Work out the finished part from the listing and answer in its coordinate system (mm). Face numbers are marked on the shaded views. A direction names the side the tool comes from. Coordinates: 2 decimals unless noted, no trailing zeros. Order: outer loops, then holes, each group sorted by start corner. A loop starts at its lowest first (then second) coordinate and runs counter-clockwise, first axis right, second up. Notation, with made-up numbers: M -34,68.25 L 2,68.25 A27 cw 2,96.25 Z; hole C -28.5,12.25 d11. An arc over 180 degrees is marked long. Use a Markdown table: item, result. Add a question column.
from build123d import *

# Parameters (mm, degrees)
F4_R     = 5
F5_DEPTH = 2.5


with BuildPart() as f2:
    # F2: sweep along a path in F0
    with BuildLine(Plane.XY) as f2_path:
        Line((0, 60), (-90, 60))
        ThreePointArc((-90, 60), (-97.0710678119, 57.0710678119), (-100, 50))
        Line((-100, 50), (-100, 0))
    # F1 (on Right) → F2 (sweep)
    with BuildSketch(Plane.YZ):
        with BuildLine():
            Line((95.0018057663, -9.8656333278), (100, -10))
            Line((100, -10), (100, 10))
            Line((100, 10), (95, 10))
            Line((95, 10), (95, 5.5))
            ThreePointArc((95, 5.5), (94.1213203436, 3.3786796564), (92, 2.5))
            Line((92, 2.5), (68, 2.5))
            ThreePointArc((68, 2.5), (65.8786796564, 3.3786796564), (65, 5.5))
            Line((65, 5.5), (65, 10))
            Line((65, 10), (60, 10))
            Line((60, 10), (60, 0))
            Line((60, 0), (60, -10))
            Line((60, -10), (65, -10))
            Line((65, -10), (65, -5.5))
            ThreePointArc((65, -5.5), (65.8786796564, -3.3786796564), (68, -2.5))
            Line((68, -2.5), (92.0018057663, -2.5))
            ThreePointArc((92.0018057663, -2.5), (94.1231261099, -3.3786796564), (95.0018057663, -5.5))
            Line((95.0018057663, -5.5), (95.0018057663, -9.8656333278))
        make_face()
    sweep(path=f2_path.line)

    # F3: F2 across plane


with BuildPart() as f2_1:
    add(f2.part)
    add(f2.part.mirror(Plane.XZ))

    # F4 (on Top) → F5 (join, symmetric)
    with BuildSketch(Plane.XY):
        with BuildLine():
            Line((-70, 100), (0, 100))
            Line((0, 100), (0, 130))
            ThreePointArc((0, 130), (-13.3277028936, 148.8541892248), (-35.5480451324, 142.5800752207))
            Line((-35.5480451324, 142.5800752207), (-70, 100))
        make_face()
        with Locations((-20, 130)):
            Circle(F4_R, mode=Mode.SUBTRACT)
        with BuildLine():
            Line((0, -130), (0, -100))
            Line((0, -100), (-70, -100))
            Line((-70, -100), (-35.5480451324, -142.5800752207))
            ThreePointArc((-35.5480451324, -142.5800752207), (-13.3277028936, -148.8541892248), (0, -130))
        make_face()
        with Locations((-20, -130)):
            Circle(F4_R, mode=Mode.SUBTRACT)
    extrude(amount=F5_DEPTH, both=True)


solid = f2_1.part
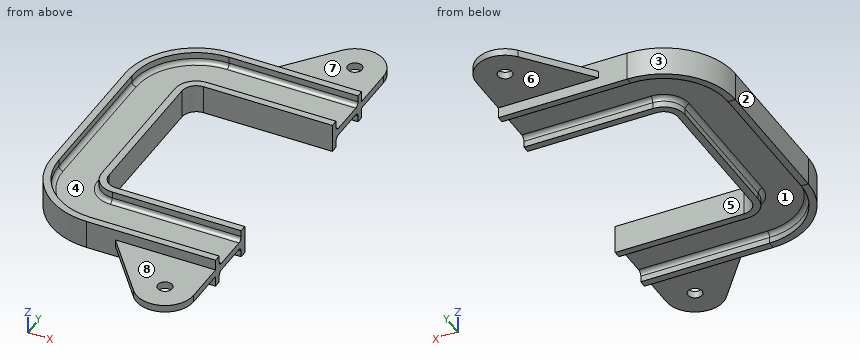
(1) Straight lines are drawn through the part: line 1 (Y direction, x = -79, z = 6); line 2 (Y direction, x = -20, z = -0.55); line 3 (X direction, y = -3.5, z = -7.75). For each, find the intervals that lie inside material, in ascending order.
(2) The mould has two halves that part along Y. Classify the marked faces 1, 2, 3 and 4: pulls with the +Y half, pulls with the -Y half, needs draft (parallel to the pull), parting line crosses it, or undercut.
(3) A cutting plane is placed at B-B on x = -20. Count the separate pieces of the cut face and the enclosed holes in it, plus the area to 3 significant figures.
(4) Which of the six approach directions +Z, -Z, +X, -X, +Y, -Y give full straight-line access (tool end or side, diameter ignored) to the marked faces 5, 6, 7 and 8?
(5) Given P1, Ø6, axis at x = -25, z = -0.5, coming from the +Y side; P2, Ø15, axis at x = -34.5, y = 121, coming from the +Z side; P3, Ø1, axis at x = -24.5, z = -2.5, coming from the +Y side, each flat-ended and moving along its own axis, determine where each tip first touches the part or whether it passes through.
(6) A cutting plane is placed at A-A on y = 23.5. Write down the section's boundary in (x, z), plus the area to 3 significant figures.
From the geometry:
| question | item | result |
|---|---|---|
| 1 | line 1 | y = -100 to -95, -65 to -60, 60 to 65, 95 to 100 |
| 1 | line 2 | y = -150 to -135, -125 to -60, 60 to 125, 135 to 150 |
| 1 | line 3 | x = -140 to -135, -105 to -100 |
| 2 | face 1 | undercut |
| 2 | face 2 | needs draft |
| 2 | face 3 | pulls with the +Y half |
| 2 | face 4 | undercut |
| 3 | separate pieces | 4 |
| 3 | enclosed holes | 0 |
| 3 | area | 1,110 mm2 |
| 4 | face 5 | +Z, -Z, +X |
| 4 | face 6 | -Z, +X, -X, +Y |
| 4 | face 7 | +Z, +X, -X, +Y |
| 4 | face 8 | +Z, +X, -X, -Y |
| 5 | P1 | stops at y = 149.9 |
| 5 | P2 | stops at z = 2.5 |
| 5 | P3 | stops at y = 149.6 |
| 6 | outline | M -140,-10 L -135,-9.87 L -135,-5.5 A3 cw -132,-2.5 L -108,-2.5 A3 cw -105,-5.5 L -105,-10 L -100,-10 L -100,10 L -105,10 L -105,5.5 A3 cw -108,2.5 L -132,2.5 A3 cw -135,5.5 L -135,10 L -140,10 Z |
| 6 | area | 357 mm2 |
